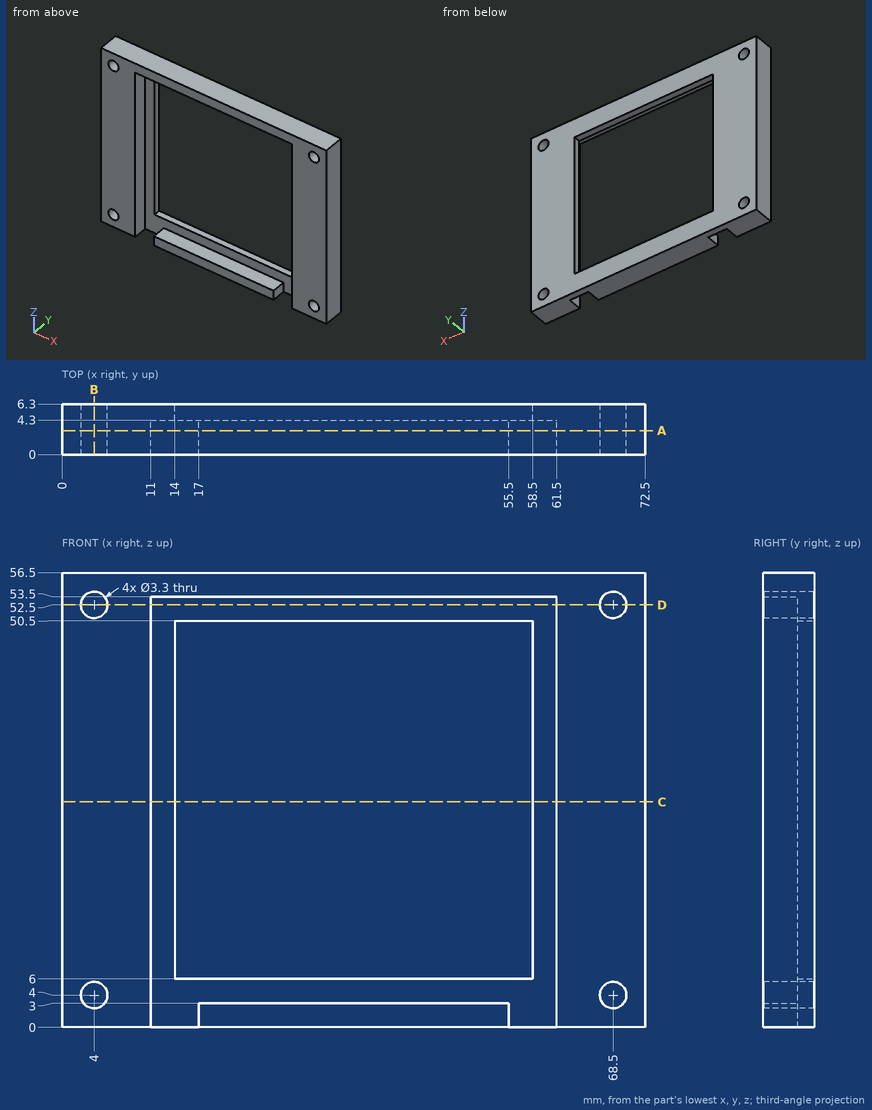
For this review, use the dimensioned drawing (mm, ordinates from the lowest corner) and the shaded views. Give positions to 0.01 mm unless a question says otherwise; leave off trailing zeros. Order: outer loops, then holes, each group sorted by start corner. A loop starts at its lowest first (then second) coordinate and runs counter-clockwise, first axis right, second up. Notation, with made-up numbers: (46.5, -22.75) - (98.5, -22.75) arc R18 ccw to (98.5, -3.75) - close; hole circle Ø8 at (-36, 0). An arc over 180 degrees is marked (long way). Use CSV: the item, a comma, the result in double quotes. Start each with the question number.
Q1. We need section A-A, the plane y = 3. Write out the cut boundary in (x, z), and give its area (3 significant figures).
Q2. We need section D-D, the plane z = 52.5. Write out the cut boundary in (x, y).
Q3. To check wall thickness, follow line 1 along X through (y, z) = (3.5, 4); line 2 along Z through (x, y) = (4, 3); line 3 along X through (y, z) = (4.5, 4). State the ranges of each line that lie inside material, in increasing order. Write a range as [from, to].
Q4. We need section B-B, the plane x = 4. Write out the cut boundary in (y, z), and give its area (3 significant figures).
Q5. We need section C-C, the plane z = 28. Write out the cut boundary in (x, y), and give its area (3 significant figures).
Outcome:
1,outline,"(0, 0) - (11, 0) - (11, 53.5) - (61.5, 53.5) - (61.5, 0) - (72.5, 0) - (72.5, 56.5) - (0, 56.5) - close; (17, 0) - (55.5, 0) - (55.5, 3) - (17, 3) - close; hole circle Ø3.3 at (4, 4); hole circle Ø3.3 at (4, 52.5); hole circle Ø3.3 at (68.5, 4); hole circle Ø3.3 at (68.5, 52.5)"
1,area,"1,480 mm^2"
2,outline,"(0, 0) - (2.35, 0) - (2.35, 6.3) - (0, 6.3) - close; (5.65, 0) - (11, 0) - (11, 4.3) - (61.5, 4.3) - (61.5, 0) - (66.85, 0) - (66.85, 6.3) - (5.65, 6.3) - close; (70.15, 0) - (72.5, 0) - (72.5, 6.3) - (70.15, 6.3) - close"
3,line 1,"x = [0, 2.35], [5.65, 11], [61.5, 66.85], [70.15, 72.5]"
3,line 2,"z = [0, 2.35], [5.65, 50.85], [54.15, 56.5]"
3,line 3,"x = [0, 2.35], [5.65, 66.85], [70.15, 72.5]"
4,outline,"(0, 0) - (6.3, 0) - (6.3, 2.35) - (0, 2.35) - close; (0, 5.65) - (6.3, 5.65) - (6.3, 50.85) - (0, 50.85) - close; (0, 54.15) - (6.3, 54.15) - (6.3, 56.5) - (0, 56.5) - close"
4,area,"314 mm^2"
5,outline,"(0, 0) - (11, 0) - (11, 4.3) - (14, 4.3) - (14, 6.3) - (0, 6.3) - close; (58.5, 4.3) - (61.5, 4.3) - (61.5, 0) - (72.5, 0) - (72.5, 6.3) - (58.5, 6.3) - close"
5,area,"151 mm^2"
